Design review of the part built by this model. Coordinates are the model's own, in mm. A direction names the side the tool comes from. Coordinates: 2 decimals unless noted, no trailing zeros. Order: outer loops, then holes, each group sorted by start corner. A loop starts at its lowest first (then second) coordinate and runs counter-clockwise, first axis right, second up. Notation, with made-up numbers: (-29, 31) -> (-4, 31) arc R21 cw to (-4, 68) -> close; hole circle Ø6 at (55, -35). An arc over 180 degrees is marked (long way). Write item = value, one per line.
```python
from build123d import *

# Parameters (mm, degrees)
SKETCH1_W           = 50.8
SKETCH1_H           = 25.4
SKETCH1_W_2         = 46.8
SKETCH1_H_2         = 21.4
BOSS_EXTRUDE1_DEPTH = 139.7
SKETCH2_W           = 21.4
SKETCH2_H           = 7.9375
CUT_EXTRUDE1_DEPTH  = 151.804144505
LPATTERN1_COUNT     = 3
LPATTERN1_PITCH     = 33.9725
LPATTERN1_COL_COUNT = 2
LPATTERN1_COL_PITCH = 38.5445
CUT_EXTRUDE2_DEPTH  = 151.804144505
LPATTERN2_COUNT     = 3
LPATTERN2_PITCH     = 50.8


with BuildPart() as part:
    # Sketch1 → Boss-Extrude1 (new body)
    with BuildSketch(Plane(origin=(0, 0, 0), x_dir=(1, 0, 0), z_dir=(0, 1, 0))):
        with Locations((25.4, 12.7)):
            Rectangle(SKETCH1_W, SKETCH1_H)
        with Locations((25.4, 12.7)):
            Rectangle(SKETCH1_W_2, SKETCH1_H_2, mode=Mode.SUBTRACT)
    extrude(amount=-BOSS_EXTRUDE1_DEPTH)

    # Sketch2 → Cut-Extrude1 (cut, through all)
    with BuildSketch(Plane(origin=(50.8, 0, 0), x_dir=(0, 0, -1), z_dir=(1, 0, 0))):
        with Locations((12.7, -69.85)):
            Rectangle(SKETCH2_W, SKETCH2_H)
    cut_extrude1 = extrude(amount=-CUT_EXTRUDE1_DEPTH, mode=Mode.SUBTRACT)

    # LPattern1: Cut-Extrude1 ×3
    with Locations(*[(0, i * LPATTERN1_PITCH, 0) for i in range(1, LPATTERN1_COUNT)]):
        add(cut_extrude1, mode=Mode.SUBTRACT)

    # LPattern1 col: Cut-Extrude1 ×2
    with Locations(*[(0, -i * LPATTERN1_COL_PITCH, 0) for i in range(1, LPATTERN1_COL_COUNT)]):
        add(cut_extrude1, mode=Mode.SUBTRACT)

    # Sketch3 → Cut-Extrude2 (cut, through all)
    with BuildSketch(Plane(origin=(0, 0, -25.4), x_dir=(-1, 0, 0), z_dir=(0, 0, -1))):
        with BuildLine():
            Line((-22.86, -21.336), (-22.86, -30.861))
            ThreePointArc((-22.86, -30.861), (-25.4, -33.401), (-27.94, -30.861))
            Line((-27.94, -30.861), (-27.94, -21.336))
            ThreePointArc((-27.94, -21.336), (-25.4, -18.796), (-22.86, -21.336))
        make_face()
    cut_extrude2 = extrude(amount=-CUT_EXTRUDE2_DEPTH, mode=Mode.SUBTRACT)

    # LPattern2: Cut-Extrude2 ×3
    with Locations(*[(0, -i * LPATTERN2_PITCH, 0) for i in range(1, LPATTERN2_COUNT)]):
        add(cut_extrude2, mode=Mode.SUBTRACT)


solid = part.part
```
(1) We need section B-B (y = -67.5). Write out the cut boundary in (x, z), and give its area (3 significant figures).
Report:
outline = (0, -25.4) -> (50.8, -25.4) -> (50.8, -23.4) -> (0, -23.4) -> close; (0, -2) -> (50.8, -2) -> (50.8, 0) -> (0, 0) -> close
area = 203 mm²
(2) Insertion check: pin 1 (0.6 mm diameter, centred on x = 49.5, z = -15.5, fed in from +Y). The pin has a flat end and moves straight along its axis. Give the tip position at first contact, or say it passes through.
Report:
pin_1 = -5.87
(3) For L1, parallel to Z at x = 43.5, y = -66; L2, parallel to X at y = -16.5, z = -2.25; L3, parallel to X at y = -28, z = -0.75, list the stretches that pass through material, from the lowest coordinate up.
Report:
L1 = -25.4 to -23.4, -2 to 0
L2 = 0 to 2, 48.8 to 50.8
L3 = 0 to 22.86, 27.94 to 50.8
(4) For faces 1 (the flat face through (25, -69, -25.4)), 2 (the flat face through (2, -53, -13)), 3 (the cylindrical face through (25.456, -120.397, -24.414)), list the 3-axis set-ups (+Z, -Z, +X, -X, +Y, -Y) from which the entire face can be reached by the end or side of a thin tool; tool diameter is ignored.
Report:
face_1 = -Z, +X, -X, +Y, -Y
face_2 = +Y, -Y
face_3 = +Z, -Z
(5) We need section A-A (x = 25.4). Give the number of separate pieces and of enclosed holes in the cut face, and give its area (3 significant figures).
Report:
separate_pieces = 8
enclosed_holes = 0
area = 384 mm²
(6) We need section D-D (x = 44). Write out the cut boundary in (y, z), and give its area (3 significant figures).
Report:
outline = (-139.7, -25.4) -> (0, -25.4) -> (0, -23.4) -> (-139.7, -23.4) -> close; (-139.7, -2) -> (0, -2) -> (0, 0) -> (-139.7, 0) -> close
area = 559 mm²
(7) The part is to be moulded in two halves that separate along X. For faces 4 (the flat face through (25, -69, 0)), 5 (the flat face through (50.8, -69, -24)), 6 (the flat face through (20, -71, -23.4)), say which applies: released by +X, released by -X, zero draft, split by the parting line, or undercut.
Report:
face_4 = zero draft
face_5 = released by +X
face_6 = undercut
